Could you check a few things on this model? Use its own coordinates, in mm. Face numbers are marked on the shaded views. Coordinates: 2 decimals unless noted, no trailing zeros. Order: outer loops, then holes, each group sorted by start corner. A loop starts at its lowest first (then second) coordinate and runs counter-clockwise, first axis right, second up. Notation, with made-up numbers: (60.5, 58) - (94.5, 58) arc R9 cw to (94.5, 71) - close; hole circle Ø3 at (-36, -26). An arc over 180 degrees is marked (long way). One line per item, written item: value.
from build123d import *

# Parameters (mm, degrees)
SKETCH1_W      = 32.004
SKETCH1_H      = 6.858
EXTRUDE1_DEPTH = 3.048
SKETCH2_W      = 0.762
SKETCH2_H      = 0.762
EXTRUDE2_DEPTH = 7.62


with BuildPart() as part:
    # Sketch1 → Extrude1 (new body)
    with BuildSketch(Plane(origin=(0, 0, 0), x_dir=(1, 0, 0), z_dir=(0, 1, 0))):
        with Locations((16.002, 3.429)):
            Rectangle(SKETCH1_W, SKETCH1_H)
    extrude(amount=EXTRUDE1_DEPTH)

    # Sketch2 → Extrude2 (add)
    with BuildSketch(Plane(origin=(0, 3.048, 0), x_dir=(1, 0, 0), z_dir=(0, 1, 0))):
        with Locations((3.429, 5.715)):
            Rectangle(SKETCH2_W, SKETCH2_H)
        with Locations((1.143, 5.715)):
            Rectangle(SKETCH2_W, SKETCH2_H)
        with Locations((5.715, 5.715)):
            Rectangle(SKETCH2_W, SKETCH2_H)
        with Locations((8.001, 5.715)):
            Rectangle(SKETCH2_W, SKETCH2_H)
        with Locations((10.287, 5.715)):
            Rectangle(SKETCH2_W, SKETCH2_H)
        with Locations((12.573, 5.715)):
            Rectangle(SKETCH2_W, SKETCH2_H)
        with Locations((14.859, 5.715)):
            Rectangle(SKETCH2_W, SKETCH2_H)
        with Locations((17.145, 5.715)):
            Rectangle(SKETCH2_W, SKETCH2_H)
        with Locations((19.431, 5.715)):
            Rectangle(SKETCH2_W, SKETCH2_H)
        with Locations((21.717, 5.715)):
            Rectangle(SKETCH2_W, SKETCH2_H)
        with Locations((24.003, 5.715)):
            Rectangle(SKETCH2_W, SKETCH2_H)
        with Locations((26.289, 5.715)):
            Rectangle(SKETCH2_W, SKETCH2_H)
        with Locations((28.575, 5.715)):
            Rectangle(SKETCH2_W, SKETCH2_H)
        with Locations((30.861, 5.715)):
            Rectangle(SKETCH2_W, SKETCH2_H)
        with Locations((1.143, 3.429)):
            Rectangle(SKETCH2_W, SKETCH2_H)
        with Locations((3.429, 3.429)):
            Rectangle(SKETCH2_W, SKETCH2_H)
        with Locations((5.715, 3.429)):
            Rectangle(SKETCH2_W, SKETCH2_H)
        with Locations((8.001, 3.429)):
            Rectangle(SKETCH2_W, SKETCH2_H)
        with Locations((10.287, 3.429)):
            Rectangle(SKETCH2_W, SKETCH2_H)
        with Locations((12.573, 3.429)):
            Rectangle(SKETCH2_W, SKETCH2_H)
        with Locations((14.859, 3.429)):
            Rectangle(SKETCH2_W, SKETCH2_H)
        with Locations((17.145, 3.429)):
            Rectangle(SKETCH2_W, SKETCH2_H)
        with Locations((19.431, 3.429)):
            Rectangle(SKETCH2_W, SKETCH2_H)
        with Locations((21.717, 3.429)):
            Rectangle(SKETCH2_W, SKETCH2_H)
        with Locations((24.003, 3.429)):
            Rectangle(SKETCH2_W, SKETCH2_H)
        with Locations((26.289, 3.429)):
            Rectangle(SKETCH2_W, SKETCH2_H)
        with Locations((28.575, 3.429)):
            Rectangle(SKETCH2_W, SKETCH2_H)
        with Locations((30.861, 3.429)):
            Rectangle(SKETCH2_W, SKETCH2_H)
        with Locations((1.143, 1.143)):
            Rectangle(SKETCH2_W, SKETCH2_H)
        with Locations((3.429, 1.143)):
            Rectangle(SKETCH2_W, SKETCH2_H)
        with Locations((5.715, 1.143)):
            Rectangle(SKETCH2_W, SKETCH2_H)
        with Locations((8.001, 1.143)):
            Rectangle(SKETCH2_W, SKETCH2_H)
        with Locations((10.287, 1.143)):
            Rectangle(SKETCH2_W, SKETCH2_H)
        with Locations((12.573, 1.143)):
            Rectangle(SKETCH2_W, SKETCH2_H)
        with Locations((14.859, 1.143)):
            Rectangle(SKETCH2_W, SKETCH2_H)
        with Locations((17.145, 1.143)):
            Rectangle(SKETCH2_W, SKETCH2_H)
        with Locations((19.431, 1.143)):
            Rectangle(SKETCH2_W, SKETCH2_H)
        with Locations((21.717, 1.143)):
            Rectangle(SKETCH2_W, SKETCH2_H)
        with Locations((24.003, 1.143)):
            Rectangle(SKETCH2_W, SKETCH2_H)
        with Locations((26.289, 1.143)):
            Rectangle(SKETCH2_W, SKETCH2_H)
        with Locations((28.575, 1.143)):
            Rectangle(SKETCH2_W, SKETCH2_H)
        with Locations((30.861, 1.143)):
            Rectangle(SKETCH2_W, SKETCH2_H)
    extrude(amount=EXTRUDE2_DEPTH)


solid = part.part
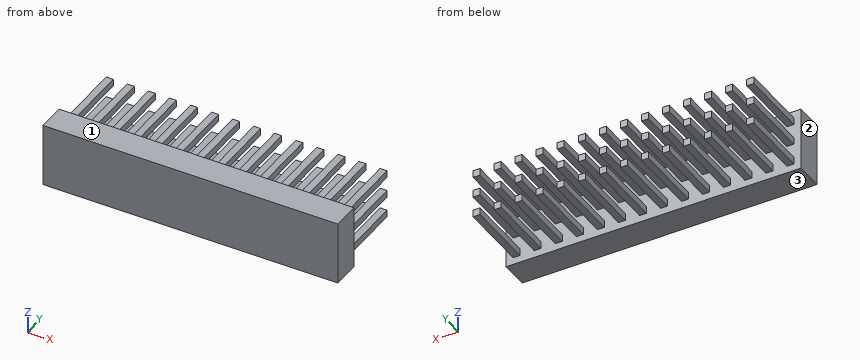
Item 1: I want a section at D-D on x = 7. Please give me the cut outline in (y, z), then the cut area to 3 significant figures.
Conclusion:
outline: (0, -6.86) - (3.05, -6.86) - (3.05, 0) - (0, 0) - close
area: 20.9 mm²
Item 2: I want a section at A-A on x = 12.5. Please give me the cut outline in (y, z), then the cut area to 3 significant figures.
Conclusion:
outline: (0, -6.86) - (3.05, -6.86) - (3.05, -6.1) - (10.67, -6.1) - (10.67, -5.33) - (3.05, -5.33) - (3.05, -3.81) - (10.67, -3.81) - (10.67, -3.05) - (3.05, -3.05) - (3.05, -1.52) - (10.67, -1.52) - (10.67, -0.76) - (3.05, -0.76) - (3.05, 0) - (0, 0) - close
area: 38.3 mm²
Item 3: If I drill on probe 1 along Y at (x, z) = (20.5, -3), over which ranges is the centre line in solid material (lowest first)?
Conclusion:
probe 1: 0 to 3.05
Item 4: I want a section at C-C on z = -4.5. Please give me the cut outline in (x, y), then the cut area to 3 significant figures.
Conclusion:
outline: (0, 0) - (32, 0) - (32, 3.05) - (0, 3.05) - close
area: 97.5 mm²
Item 5: Thinking about a two-plate mould opening in Z: for the marked faces 1, 2 and 3, which applies, pulls with the +Z half, pulls with the -Z half, needs draft (parallel to the pull), parting line crosses it, or undercut?
Conclusion:
face 1: pulls with the +Z half
face 2: needs draft
face 3: pulls with the -Z half
Item 6: I want a section at B-B on y = 7.5. Give the number of separate pieces and of enclosed holes in the cut face, then the cut area to 3 significant figures.
Conclusion:
separate pieces: 42
enclosed holes: 0
area: 24.4 mm²
Item 7: I'm going to push flat-ended pins straight in: pin 1 Ø0.6 at (x, y) = (5.5, 7) entering from -Z; pin 2 Ø0.6 at (x, y) = (10.5, 5) entering from +Z; pin 3 Ø3 at (y, z) = (5, -1.5) entering from -X; pin 4 Ø3.5 at (x, z) = (15.5, -2) entering from +Y. Where does each tip first touch, or does it pass through?
Conclusion:
pin 1: z = -6.1
pin 2: z = -0.76
pin 3: x = 0.76
pin 4: y = 10.67
